```python
from build123d import *

# Parameters (mm, degrees)
SKETCH1_W            = 11.0236
SKETCH1_H            = 1.905
BOSS_EXTRUDE1_START  = 2.54
SKETCH4_R            = 9.5504
BOSS_EXTRUDE1_DEPTH  = 2.54
M3_CLEARANCE_HOLE1_D = 3.2
BOSS_EXTRUDE4_START  = 22.225
BOSS_EXTRUDE4_DEPTH  = 22.225
FILLET1_R            = 2.54
SKETCH8_R            = 4.445
SKETCH8_R_2          = 1.3890625
BOSS_EXTRUDE5_DEPTH  = 19.685
FILLET3_R            = 2.54
FILLET4_R            = 2.54


with BuildPart() as part:
    # Sketch1 → Revolve1 (revolve)
    with BuildSketch(Plane.XY, mode=Mode.PRIVATE) as revolve1_sk:
        with Locations((-15.0622, -0.9525)):
            Rectangle(SKETCH1_W, SKETCH1_H)
    revolve(revolve1_sk.sketch.rotate(Axis((0, 0, 0), (0, 1, 0)), 270), axis=Axis((0, 0, 0), (0, 1, 0)))

    # Sketch4 → Boss-Extrude1 (add)
    with BuildSketch(Plane(origin=(0, 0, 0), x_dir=(1, 0, 0), z_dir=(0, 1, 0)).offset(BOSS_EXTRUDE1_START)):
        with BuildLine():
            Line((-24.13, -67.31), (24.13, -67.31))
            ThreePointArc((24.13, -67.31), (31.314204897, -64.334204897), (34.29, -57.15))
            Line((34.29, -57.15), (34.29, 24.13))
            ThreePointArc((34.29, 24.13), (31.314204897, 31.314204897), (24.13, 34.29))
            Line((24.13, 34.29), (-24.13, 34.29))
            ThreePointArc((-24.13, 34.29), (-31.314204897, 31.314204897), (-34.29, 24.13))
            Line((-34.29, 24.13), (-34.29, -57.15))
            ThreePointArc((-34.29, -57.15), (-31.314204897, -64.334204897), (-24.13, -67.31))
        make_face()
        Circle(SKETCH4_R, mode=Mode.SUBTRACT)
    extrude(amount=-BOSS_EXTRUDE1_DEPTH)

    # M3 Clearance Hole1 (through all)
    with Locations(Plane(origin=(0, 2.54, 0), x_dir=(1, 0, 0), z_dir=(0, 1, 0))):
        with Locations((-13.858138511, -8.001), (-16.002, 0), (-13.858138511, 8.001), (-8.001, 13.858138511), (0, 16.002), (8.001, 13.858138511), (13.858138511, 8.001), (16.002, 0), (13.858138511, -8.001), (8.001, -13.858138511), (0, -16.002), (-8.001, -13.858138511)):
            Hole(M3_CLEARANCE_HOLE1_D / 2)

    # Sketch6 → Boss-Extrude4 (add)
    with BuildSketch(Plane(origin=(0, 2.54, 0), x_dir=(1, 0, 0), z_dir=(0, 1, 0)).offset(BOSS_EXTRUDE4_START)):
        with BuildLine():
            Line((24.13, 34.29), (-24.13, 34.29))
            ThreePointArc((-24.13, 34.29), (-31.314204897, 31.314204897), (-34.29, 24.13))
            Line((-34.29, 24.13), (-34.29, -57.15))
            ThreePointArc((-34.29, -57.15), (-31.314204897, -64.334204897), (-24.13, -67.31))
            Line((-24.13, -67.31), (24.13, -67.31))
            ThreePointArc((24.13, -67.31), (31.314204897, -64.334204897), (34.29, -57.15))
            Line((34.29, -57.15), (34.29, 24.13))
            ThreePointArc((34.29, 24.13), (31.314204897, 31.314204897), (24.13, 34.29))
        make_face()
        with BuildLine():
            Line((24.13, 31.75), (-24.13, 31.75))
            ThreePointArc((-24.13, 31.75), (-29.518153673, 29.518153673), (-31.75, 24.13))
            Line((-31.75, 24.13), (-31.75, -57.15))
            ThreePointArc((-31.75, -57.15), (-29.518153673, -62.538153673), (-24.13, -64.77))
            Line((-24.13, -64.77), (24.13, -64.77))
            ThreePointArc((24.13, -64.77), (29.518153673, -62.538153673), (31.75, -57.15))
            Line((31.75, -57.15), (31.75, 24.13))
            ThreePointArc((31.75, 24.13), (29.518153673, 29.518153673), (24.13, 31.75))
        make_face(mode=Mode.SUBTRACT)
    extrude(amount=-BOSS_EXTRUDE4_DEPTH)

    # Fillet1
    fillet1_edges = [part.edges().sort_by_distance(p)[0] for p in [
        (-31.314204897, 0, 64.334204897),
        (0, 0, 67.31),
        (31.314204897, 0, 64.334204897),
        (34.29, 0, 16.51),
        (31.314204897, 0, -31.314204897),
        (0, 0, -34.29),
        (-31.314204897, 0, -31.314204897),
        (-34.29, 0, 16.51),
    ]]
    fillet(fillet1_edges, radius=FILLET1_R)

    # Sketch8 → Boss-Extrude5 (add)
    # profile 1 of 4: a face of its own
    with BuildSketch(Plane(origin=(0, 2.54, 0), x_dir=(1, 0, 0), z_dir=(0, 1, 0))):
        with Locations((-27.722102448, -60.742102448)):
            Circle(SKETCH8_R)
        with Locations(Location((-27.722102448, -60.742102448, 0), (0, 0, 270))):
            Circle(SKETCH8_R_2, mode=Mode.SUBTRACT)
    # profile 2 of 4: a face of its own
    with BuildSketch(Plane(origin=(0, 2.54, 0), x_dir=(1, 0, 0), z_dir=(0, 1, 0))):
        with Locations((27.722102448, -60.742102448)):
            Circle(SKETCH8_R)
        with Locations(Location((27.722102448, -60.742102448, 0), (0, 0, 270))):
            Circle(SKETCH8_R_2, mode=Mode.SUBTRACT)
    # profile 3 of 4: a face of its own
    with BuildSketch(Plane(origin=(0, 2.54, 0), x_dir=(1, 0, 0), z_dir=(0, 1, 0))):
        with Locations((27.722102448, 27.722102448)):
            Circle(SKETCH8_R)
        with Locations(Location((27.722102448, 27.722102448, 0), (0, 0, 270))):
            Circle(SKETCH8_R_2, mode=Mode.SUBTRACT)
    # profile 4 of 4: a face of its own
    with BuildSketch(Plane(origin=(0, 2.54, 0), x_dir=(1, 0, 0), z_dir=(0, 1, 0))):
        with Locations((-27.722102448, 27.722102448)):
            Circle(SKETCH8_R)
        with Locations(Location((-27.722102448, 27.722102448, 0), (0, 0, 270))):
            Circle(SKETCH8_R_2, mode=Mode.SUBTRACT)
    extrude(amount=BOSS_EXTRUDE5_DEPTH)

    # Fillet3
    # the kernel refuses this fillet: 2.54 mm, written as the material it adds along each edge
    with BuildSketch(Plane(origin=(25.571770391, 2.54, 64.632359129), x_dir=(-0.5973974080073474, 0, -0.8019453453360166), z_dir=(0, 1, 0)), Plane(origin=(31.612359129, 2.54, -25.571770391), x_dir=(-0.8019453453360167, 0, 0.5973974080073472), z_dir=(0, 1, 0)), Plane(origin=(-25.571770391, 2.54, -31.612359129), x_dir=(0.5973974080073424, 0, 0.8019453453360202), z_dir=(0, 1, 0)), Plane(origin=(-31.612359129, 2.54, 58.591770391), x_dir=(0.8019453453360194, 0, -0.5973974080073438), z_dir=(0, 1, 0))) as fillet3_piece_1:
        with BuildLine():
            CenterArc((4.719009703, 2.313416024), FILLET3_R, 143.316272758, 102.298995101)
            Line((2.682068526, 3.83080544), (2.478374408, 3.982544382))
            ThreePointArc((2.478374408, 3.982544382), (0.547235321, 1.390186295), (-0.228725099, 0.110457363))
            Line((-0.228725099, 0.110457363), (0.104866882, -0.231341602))
            ThreePointArc((0.104866882, -0.231341602), (1.83517044, 0.142521958), (3.565473998, -0.231341602))
            Line((3.565473998, -0.231341602), (3.67034088, 0))
        make_face()
    extrude(amount=19.685)
    with BuildSketch(Plane(origin=(31.612359129, 2.54, 58.591770391), x_dir=(-0.8019453453360176, 0, -0.5973974080073462), z_dir=(0, 1, 0)), Plane(origin=(25.571770391, 2.54, -31.612359129), x_dir=(-0.5973974080073442, 0, 0.801945345336019), z_dir=(0, 1, 0)), Plane(origin=(-31.612359129, 2.54, -25.571770391), x_dir=(0.8019453453360176, 0, 0.5973974080073461), z_dir=(0, 1, 0)), Plane(origin=(-25.571770391, 2.54, 64.632359129), x_dir=(0.5973974080073453, 0, -0.8019453453360182), z_dir=(0, 1, 0))) as fillet3_piece_2:
        with BuildLine():
            CenterArc((4.719009703, -2.313416024), FILLET3_R, 114.384732141, 102.298995101)
            Line((2.682068526, -3.83080544), (2.478374408, -3.982544382))
            ThreePointArc((2.478374408, -3.982544382), (0.547235321, -1.390186295), (-0.228725099, -0.110457363))
            Line((-0.228725099, -0.110457363), (0.104866882, 0.231341602))
            ThreePointArc((0.104866882, 0.231341602), (1.83517044, -0.142521958), (3.565473998, 0.231341602))
            Line((3.565473998, 0.231341602), (3.67034088, 0))
        make_face()
    extrude(amount=19.685)

    # Fillet4
    fillet4_edges = [part.edges().sort_by_distance(p)[0] for p in [
        (0, 2.54, 64.77),
        (-24.579012806, 2.54, -24.579012806),
        (-31.75, 2.54, 16.51),
        (-24.579012806, 2.54, 57.599012806),
        (24.579012806, 2.54, 57.599012806),
        (31.75, 2.54, 16.51),
        (24.579012806, 2.54, -24.579012806),
        (0, 2.54, -31.75),
        (-22.875527809, 2.54, 63.823317877),
        (-30.803317877, 2.54, 55.895527809),
        (-22.875527809, 2.54, -30.803317877),
        (-30.803317877, 2.54, -22.875527809),
        (30.803317877, 2.54, -22.875527809),
        (22.875527809, 2.54, -30.803317877),
        (30.803317877, 2.54, 55.895527809),
        (22.875527809, 2.54, 63.823317877),
    ]]
    fillet(fillet4_edges, radius=FILLET4_R)


solid = part.part
```
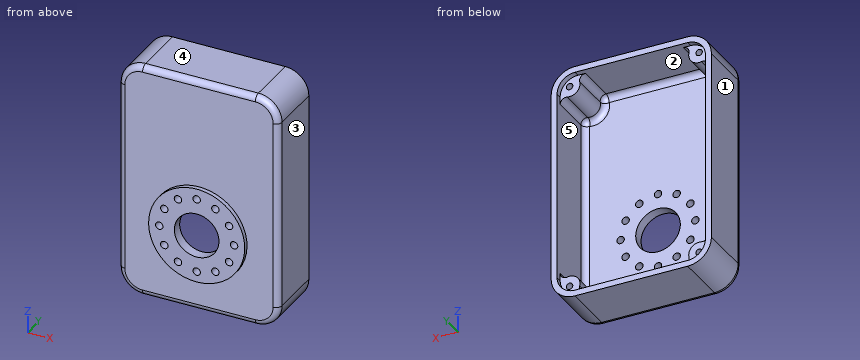
Input: part model. Units: mm. Frame: model coordinates. Face numbers are marked on the shaded views. A direction names the side the tool comes from. Round coordinates to 2 decimals unless told otherwise and drop trailing zeros. Loops run counter-clockwise (first coordinate to the right, second up) from the corner with the lowest first, then second, coordinate; pieces in that order, holes last. Notation, with made-up numbers: M 33.5,63.25 L 71.5,63.25 A18 ccw 71.5,90.25 Z; hole C 89.5,-16.5 d10. An arc over 180 degrees is marked long. Answer in a Markdown table with one row per item. Add a question column.
1. Section A-A (x = 0). Output: boundary loops of the cut face in (y, z) (3 decimals).
2. Section C-C (y = 7.25). Output: boundary loops of the cut face in (x, z) (3 decimals), and give its area (3 significant figures).
3. Section B-B (z = 0). Output: boundary loops of the cut face in (x, y) (3 decimals), and give its area (3 significant figures).
4. Mould query, pull axis X, two halves, no side actions, for the marked faces 1, 2 and 3. Classes: released by +X, released by -X, zero draft, split by the parting line, or undercut.
5. Contact query for flat-ended pins moving along their axis: pin 1 (4 mm diameter, centred on x = 13.86, z = -8, fed in from -Y) (3 decimals); pin 2 (3 mm diameter, centred on x = -14.5, z = 37.5, fed in from -Y); pin 3 (1.7 mm diameter, centred on x = 27.72, z = -27.72, fed in from +Y); pin 4 (5.5 mm diameter, centred on x = -27, z = 57, fed in from +Y) (3 decimals). Output: stop coordinate, or through.
6. Ray query, probe 1 along Z at (x, y) = (15.5, 8.5); probe 2 along X at (y, z) = (5, 26); probe 3 along Z at (x, y) = (28, 19.5). Return the intervals inside material, ascending.
7. Set-up query: the marked faces 4 and 5. Return all of +Z, -Z, +X, -X, +Y, -Y with unobstructed straight access to the full face (end or side cutting, diameter ignored); none if empty.
8. Section D-D (z = 52). Output: boundary loops of the cut face in (x, y) (3 decimals), and give its area (3 significant figures).
Values follow:
| question | item | result |
|---|---|---|
| 1 | outline | M -1.905,-20.574 L 0,-20.574 L 0,-31.75 A2.54 ccw 2.54,-34.29 L 24.765,-34.29 L 24.765,-31.75 L 5.08,-31.75 A2.54 cw 2.54,-29.21 L 2.54,-17.602 L -1.905,-17.602 Z; M -1.905,-14.402 L 2.54,-14.402 L 2.54,-9.55 L -1.905,-9.55 Z; M -1.905,9.55 L 2.54,9.55 L 2.54,14.402 L -1.905,14.402 Z; M -1.905,17.602 L 2.54,17.602 L 2.54,62.23 A2.54 cw 5.08,64.77 L 24.765,64.77 L 24.765,67.31 L 2.54,67.31 A2.54 ccw 0,64.77 L 0,20.574 L -1.905,20.574 Z |
| 2 | outline | M -34.29,-24.13 A10.16 ccw -24.13,-34.29 L 24.13,-34.29 A10.16 ccw 34.29,-24.13 L 34.29,57.15 A10.16 ccw 24.13,67.31 L -24.13,67.31 A10.16 ccw -34.29,57.15 Z; hole M -31.75,-20.897 A2.54 ccw -28.669,-23.379 A4.445 cw -23.379,-28.669 A2.54 ccw -20.897,-31.75 L 20.897,-31.75 A2.54 ccw 23.379,-28.669 A4.445 cw 28.669,-23.379 A2.54 ccw 31.75,-20.897 L 31.75,53.917 A2.54 ccw 28.669,56.399 A4.445 cw 23.379,61.689 A2.54 ccw 20.897,64.77 L -20.897,64.77 A2.54 ccw -23.379,61.689 A4.445 cw -28.669,56.399 A2.54 ccw -31.75,53.917 Z; hole C -27.722,-27.722 d2.778; hole C -27.722,60.742 d2.778; hole C 27.722,-27.722 d2.778; hole C 27.722,60.742 d2.778 |
| 2 | area | 1,000 mm^2 |
| 3 | outline | M -34.29,2.54 A2.54 ccw -31.75,0 L -20.574,0 L -20.574,-1.905 L -17.602,-1.905 L -17.602,2.54 L -29.21,2.54 A2.54 cw -31.75,5.08 L -31.75,24.765 L -34.29,24.765 Z; M -14.402,-1.905 L -9.55,-1.905 L -9.55,2.54 L -14.402,2.54 Z; M 9.55,-1.905 L 14.402,-1.905 L 14.402,2.54 L 9.55,2.54 Z; M 17.602,-1.905 L 20.574,-1.905 L 20.574,0 L 31.75,0 A2.54 ccw 34.29,2.54 L 34.29,24.765 L 31.75,24.765 L 31.75,5.08 A2.54 cw 29.21,2.54 L 17.602,2.54 Z |
| 3 | area | 252 mm^2 |
| 4 | face 1 | released by -X |
| 4 | face 2 | undercut |
| 4 | face 3 | released by +X |
| 5 | pin 1 | y = -1.905 |
| 5 | pin 2 | y = 0 |
| 5 | pin 3 | y = 2.54 |
| 5 | pin 4 | y = 22.225 |
| 6 | probe 1 | -34.29 to -31.75, 64.77 to 67.31 |
| 6 | probe 2 | -34.29 to -31.75, 31.75 to 34.29 |
| 6 | probe 3 | -33.52 to -29.08, -26.36 to -23.29, 56.31 to 59.38, 62.1 to 66.54 |
| 7 | face 4 | +Z, +X, -X, +Y, -Y |
| 7 | face 5 | +Y |
| 8 | outline | M -34.29,2.54 A2.54 ccw -31.75,0 L 31.75,0 A2.54 ccw 34.29,2.54 L 34.29,24.765 L 31.75,24.765 L 31.75,5.08 A2.54 cw 29.21,2.54 L -29.21,2.54 A2.54 cw -31.75,5.08 L -31.75,24.765 L -34.29,24.765 Z |
| 8 | area | 287 mm^2 |
